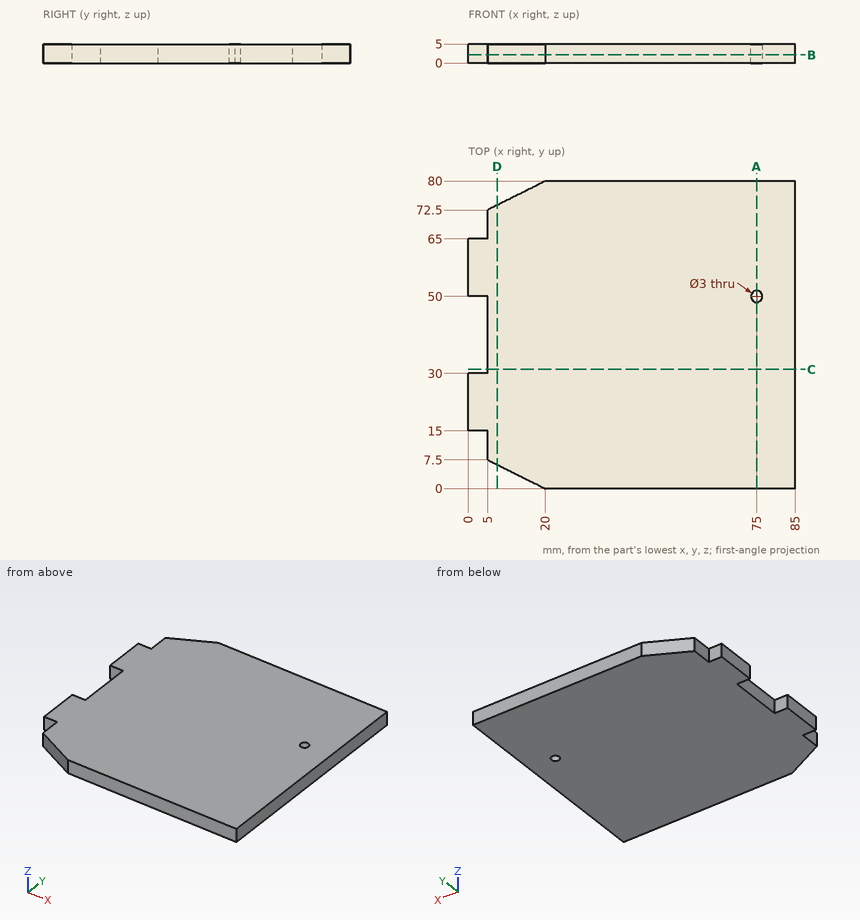
Check sheet for the drawn part. Datum: minimum x, y, z corner. Units: mm. Give positions to 0.01 mm unless a question says otherwise; leave off trailing zeros. Write each loop counter-clockwise with the first axis right and the second up, starting at its lowest first coordinate (ties: lowest second). Pieces come first, ordered by that corner, then holes.
(1) Cross-section at D-D (x = 7.5). Enter the section's corners in (y, z), plus the area to 4 significant figures.
(2) Cross-section at A-A (x = 75). Enter the section's corners in (y, z).
(3) Cross-section at B-B (z = 2.15). Enter the section's corners in (x, y), plus the area to 3 significant figures.
(4) Cross-section at C-C (y = 31). Enter the section's corners in (x, z), plus the area to 3 significant figures.
(5) Gauge pin test, flat ends, axial feed: pin 1 (1.5 mm diameter, centred on y = 35.5, z = 1.5, fed in from -X); pin 2 (2.5 mm diameter, centred on x = 2, z = 2, fed in from +Y). Record the tip position at first contact, or that the pin passes through.
(6) Material ranges on line 1 (Y direction, x = 75, z = 2.75); line 2 (X direction, y = 12.5, z = 1.25); line 3 (X direction, y = 77, z = 1.25), recorded low to high.
Worked out:
1. outline: (6.25, 0) - (73.75, 0) - (73.75, 5) - (6.25, 5) - close
1. area: 337.5 mm2
2. outline: (0, 0) - (48.5, 0) - (48.5, 5) - (0, 5) - close; (51.5, 0) - (80, 0) - (80, 5) - (51.5, 5) - close
3. outline: (0, 15) - (5, 15) - (5, 7.5) - (20, 0) - (85, 0) - (85, 80) - (20, 80) - (5, 72.5) - (5, 65) - (0, 65) - (0, 50) - (5, 50) - (5, 30) - (0, 30) - close; hole circle Ø3 at (75, 50)
3. area: 6,430 mm2
4. outline: (5, 0) - (85, 0) - (85, 5) - (5, 5) - close
4. area: 400 mm2
5. pin 1: stops at x = 5
5. pin 2: stops at y = 65
6. line 1: y = 0 to 48.5, 51.5 to 80
6. line 2: x = 5 to 85
6. line 3: x = 14 to 85
